from build123d import *

# Parameters (mm, degrees)
SKETCH1_R           = 4.5
SKETCH1_W           = 9
SKETCH1_H           = 27.94
BOSS_EXTRUDE1_DEPTH = 2
SKETCH2_R           = 1.6
CUT_EXTRUDE1_DEPTH  = 10


with BuildPart() as part:
    # Sketch1 → Boss-Extrude1 (new body)
    with BuildSketch(Plane(origin=(0, 0, 0), x_dir=(1, 0, 0), z_dir=(0, 1, 0))):
        Circle(SKETCH1_R)
        with Locations((0, -27.94)):
            Circle(SKETCH1_R)
        with Locations((0, -13.97)):
            Rectangle(SKETCH1_W, SKETCH1_H)
    extrude(amount=BOSS_EXTRUDE1_DEPTH)

    # Sketch2 → Cut-Extrude1 (cut)
    with BuildSketch(Plane(origin=(0, 2, 0), x_dir=(1, 0, 0), z_dir=(0, 1, 0))):
        with Locations(Location((0, 0, 0), (0, 0, 270))):
            Circle(SKETCH2_R)
        with Locations(Location((0, -27.94, 0), (0, 0, 270))):
            Circle(SKETCH2_R)
    extrude(amount=-CUT_EXTRUDE1_DEPTH, mode=Mode.SUBTRACT)


solid = part.part
Source: CAD feature listing. Evaluate the final solid. Frame: model axes, mm. Round coordinates to 2 decimals unless told otherwise and drop trailing zeros. Loops run counter-clockwise (first coordinate to the right, second up) from the corner with the lowest first, then second, coordinate; pieces in that order, holes last. Notation, with made-up numbers: (-8.5, 24) -> (40.5, 24) arc R14 ccw to (40.5, 39) -> close; hole circle Ø11 at (-20.75, 83). An arc over 180 degrees is marked (long way). Answer as a JSON object with one key per item and string values. Group by question number.
Q1. Section query A-A (x = -1.25). Output: boundary loops of the cut face in (y, z).
Q2. Section query B-B (y = 0.6). Output: boundary loops of the cut face in (x, z), plus the area to 3 significant figures.
Q3. Mould query, pull axis Z, two halves, no side actions, for faces 1 (the cylindrical face through (0.1, 1, -4.5)), 2 (the flat face through (0, 0, 14)), 3 (the cylindrical face through (1.08, 1.01, 26.76)). Classes: pulls with the +Z half, pulls with the -Z half, needs draft (parallel to the pull), parting line crosses it, or undercut.
Q4. Ray query, line 1 (Z direction, x = -0.75, y = 0.2); line 2 (X direction, y = 1.2, z = 0); line 3 (Z direction, x = 1.25, y = 1.6). Return the intervals inside material, ascending. Write a range as from..to.
Q5. Section query C-C (x = 2.25). Output: boundary loops of the cut face in (y, z), plus the area to 3 significant figures.
Completed:
{
 "1": {"outline": "(0, -4.32) -> (2, -4.32) -> (2, -1) -> (0, -1) -> close; (0, 1) -> (2, 1) -> (2, 26.94) -> (0, 26.94) -> close; (0, 28.94) -> (2, 28.94) -> (2, 32.26) -> (0, 32.26) -> close"},
 "2": {"outline": "(-4.5, 0) arc R4.5 ccw to (4.5, 0) -> (4.5, 27.94) arc R4.5 ccw to (-4.5, 27.94) -> close; hole circle Ø3.2 at (0, 0); hole circle Ø3.2 at (0, 27.94)", "area": "299 mm²"},
 "3": {"face 1": "pulls with the -Z half", "face 2": "needs draft", "face 3": "undercut"},
 "4": {"line 1": "-4.44..-1.41, 1.41..26.53, 29.35..32.38", "line 2": "-4.5..-1.6, 1.6..4.5", "line 3": "-4.32..-1, 1..26.94, 28.94..32.26"},
 "5": {"outline": "(0, -3.9) -> (2, -3.9) -> (2, 31.84) -> (0, 31.84) -> close", "area": "71.5 mm²"}
}
